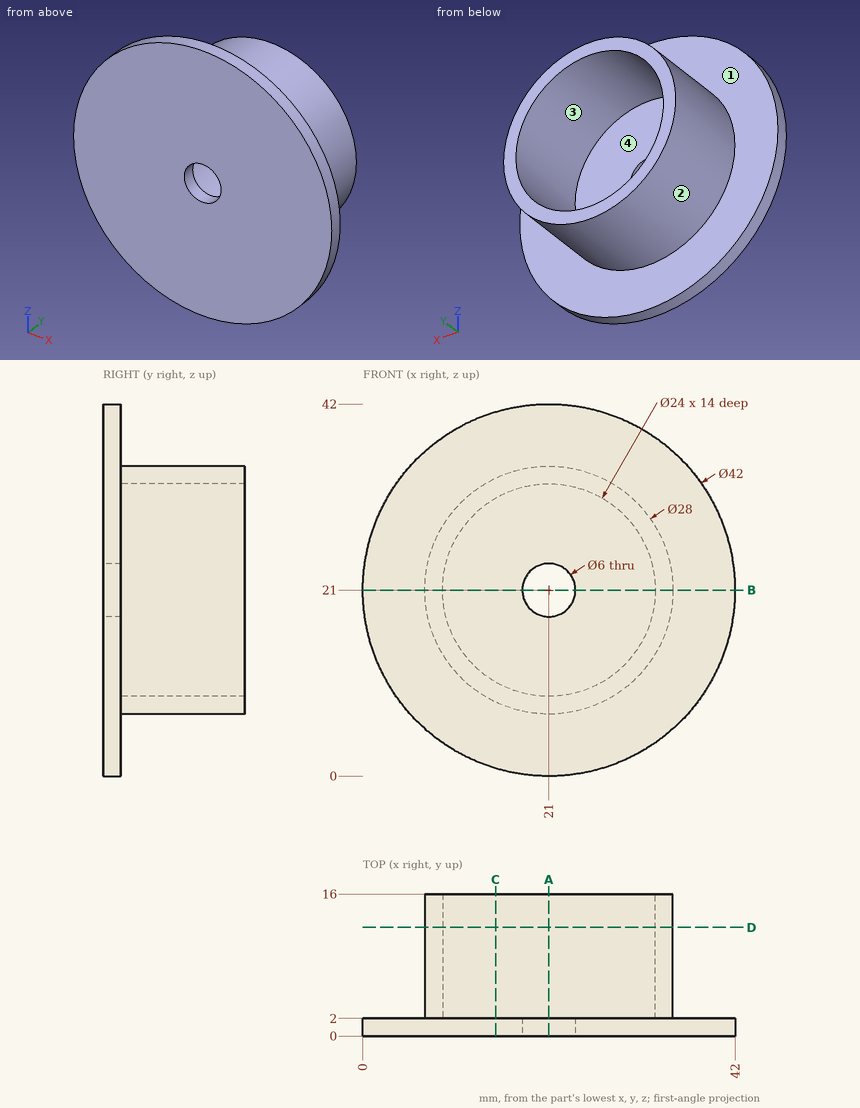
Input: dimensioned drawing with shaded views. Units: mm. Origin: part minimum x, y, z. Give positions to 0.01 mm unless a question says otherwise; leave off trailing zeros. Write each loop counter-clockwise with the first axis right and the second up, starting at its lowest first coordinate (ties: lowest second). Pieces come first, ordered by that corner, then holes. Notation, with made-up numbers: M -12,74.25 L 26,74.25 A22 cw 26,100.25 Z; hole C 16.25,2 d2. An arc over 180 degrees is marked long. Return JSON: item names as keys, results as strings. Group by question number.
1) Cut plane D-D, the plane y = 12.25. Output: boundary loops of the cut face in (x, z), plus the area to 3 significant figures.
2) Cut plane B-B, the plane z = 21. Output: boundary loops of the cut face in (x, y).
3) Pull-direction query (Z, two-part tool) for the marked faces 1, 2, 3 and 4; classes: pulls with the +Z half, pulls with the -Z half, needs draft (parallel to the pull), parting line crosses it, or undercut.
4) Cut plane A-A, the plane x = 21. Output: boundary loops of the cut face in (y, z), plus the area to 3 significant figures.
5) Pin query (flat end, axial travel): P1, Ø4, axis at x = 21, y = 14, coming from the -Z side; P2, Ø9.5, axis at x = 21, z = 21, coming from the +Y side; P3, Ø1.5, axis at x = 31, y = 13.5, coming from the +Z side; P4, Ø10, axis at x = 15, z = 29, coming from the +Y side. Return the tip coordinate at first contact, or that it passes through.
6) Cut plane C-C, the plane x = 15. Output: boundary loops of the cut face in (y, z), plus the area to 3 significant figures.
7) Material intervals for line 1 along Z through (x, y) = (21, 8); line 2 along X through (y, z) = (0.9, 21), sorted ascending. Write a range as [from, to].
Recorded:
{
 "1": {"outline": "C 21,21 d28; hole C 21,21 d24", "area": "163 mm²"},
 "2": {"outline": "M 0,0 L 18,0 L 18,2 L 9,2 L 9,16 L 7,16 L 7,2 L 0,2 Z; M 24,0 L 42,0 L 42,2 L 35,2 L 35,16 L 33,16 L 33,2 L 24,2 Z"},
 "3": {"face 1": "needs draft", "face 2": "parting line crosses it", "face 3": "undercut", "face 4": "undercut"},
 "4": {"outline": "M 0,0 L 2,0 L 2,7 L 16,7 L 16,9 L 2,9 L 2,18 L 0,18 Z; M 0,24 L 2,24 L 2,33 L 16,33 L 16,35 L 2,35 L 2,42 L 0,42 Z", "area": "128 mm²"},
 "5": {"P1": "stops at z = 7", "P2": "stops at y = 2", "P3": "stops at z = 31.51", "P4": "stops at y = 16"},
 "6": {"outline": "M 0,0.88 L 2,0.88 L 2,8.35 L 16,8.35 L 16,10.61 L 2,10.61 L 2,31.39 L 16,31.39 L 16,33.65 L 2,33.65 L 2,41.12 L 0,41.12 Z", "area": "144 mm²"},
 "7": {"line 1": "z = [7, 9], [33, 35]", "line 2": "x = [0, 18], [24, 42]"}
}
